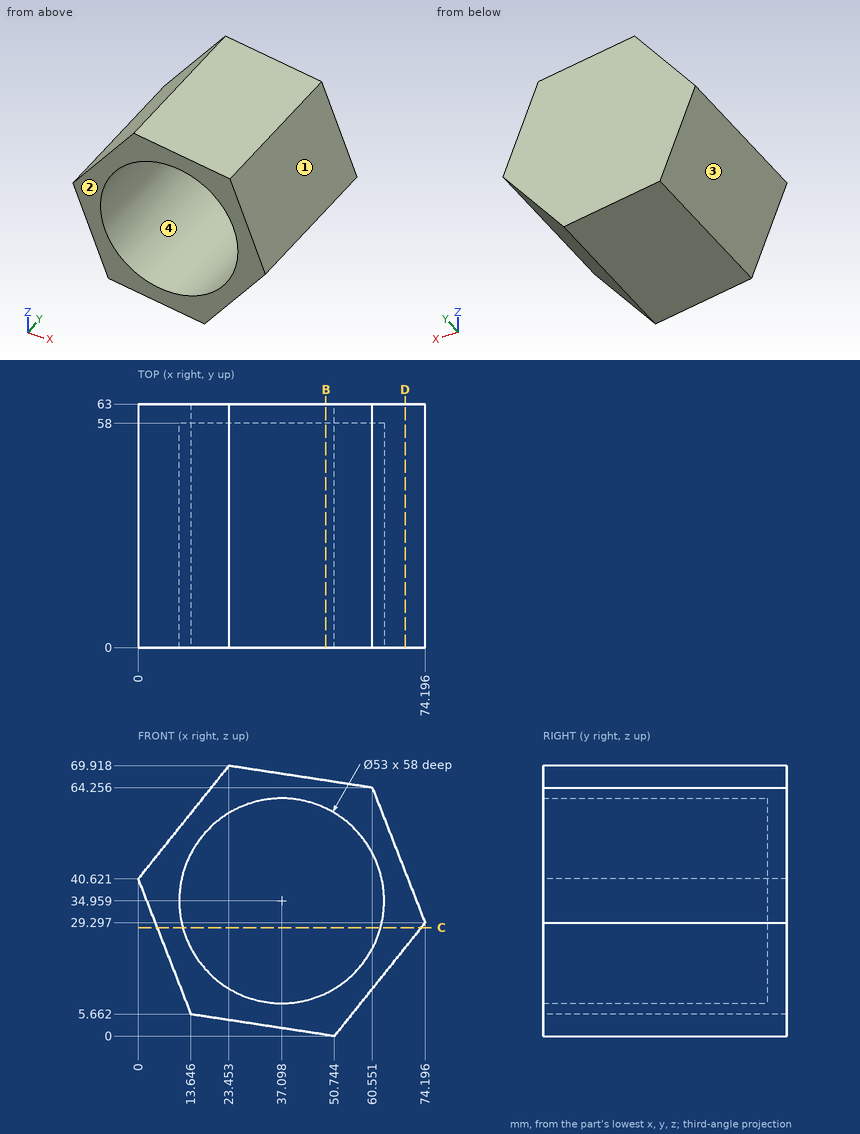
Here's the drawing with two shaded views (mm, measured from the low corner). I have some questions. Round coordinates to 2 decimals unless told otherwise and drop trailing zeros. Order: outer loops, then holes, each group sorted by start corner. A loop starts at its lowest first (then second) coordinate and runs counter-clockwise, first axis right, second up. Notation, with made-up numbers: (-26, 69) -> (5, 69) arc R25 ccw to (5, 107) -> close; hole circle Ø2 at (22.25, 31). An arc over 180 degrees is marked (long way). Use a Markdown table: item, result. Add a question column.
(1) Suppose I cut it at C-C, the plane z = 28. Please give me the cut outline in (x, y), and give its area (3 significant figures).
(2) For pin 1 Ø5 at (x, y) = (20, 11.5) entering from -Z; pin 2 Ø12 at (x, y) = (57, 39) entering from -Z; pin 3 Ø1.5 at (x, y) = (39.5, 25.5) entering from -Z, each with a flat end and sliding along its axis, tell me the tip position at first contact or that it passes through.
(3) If we mould it in two halves opening along Z, with no side actions, what happens to the marked faces 1, 2, 3 and 4? For each: released by +Z, released by -Z, zero draft, split by the parting line, or undercut.
(4) Suppose I cut it at D-D, the plane x = 69. Please give me the cut outline in (y, z) (1 decimal).
(5) Suppose I cut it at B-B, the plane x = 48.5. Please give me the cut outline in (y, z) (1 decimal).
(6) I need wall thicknesses on line 1 along Z through (x, y) = (29, 37.5); line 2 along Y through (x, z) = (30, 18.5); line 3 along Z through (x, y) = (16, 40.5) (1 decimal). Which ranges of each line are inside material? Lowest first, please.
Verdict:
| question | item | result |
|---|---|---|
| 1 | outline | (4.93, 0) -> (11.53, 0) -> (11.53, 58) -> (62.67, 58) -> (62.67, 0) -> (73.16, 0) -> (73.16, 63) -> (4.93, 63) -> close |
| 1 | area | 1,330 mm2 |
| 2 | pin 1 | z = 4.31 |
| 2 | pin 2 | z = 0.32 |
| 2 | pin 3 | z = 1.6 |
| 3 | face 1 | released by +Z |
| 3 | face 2 | zero draft |
| 3 | face 3 | released by -Z |
| 3 | face 4 | undercut |
| 4 | outline | (0, 22.8) -> (63, 22.8) -> (63, 42.6) -> (0, 42.6) -> close |
| 5 | outline | (0, 0.3) -> (63, 0.3) -> (63, 66.1) -> (0, 66.1) -> (0, 58.9) -> (58, 58.9) -> (58, 11) -> (0, 11) -> close |
| 6 | line 1 | 3.32 to 9.73, 60.19 to 69.07 |
| 6 | line 2 | 58 to 63 |
| 6 | line 3 | 5.3 to 18.9, 51 to 60.6 |
